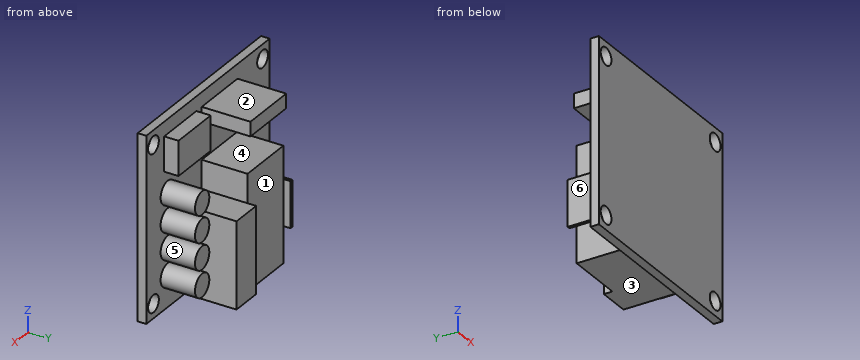
```python
from build123d import *

# Parameters (mm, degrees)
SKETCH_1_W      = 34.5
SKETCH_1_H      = 32
SKETCH_1_R      = 1.5
SKETCH_1_W_2    = 10
SKETCH_1_H_2    = 2.5
SKETCH_1_W_3    = 9
SKETCH_1_H_3    = 6
SKETCH_1_R_2    = 2
SKETCH_1_W_4    = 2.5
SKETCH_1_H_4    = 10
SKETCH_1_W_5    = 0.5
SKETCH_1_H_5    = 8
SKETCH_1_H_6    = 20
SKETCH_1_W_6    = 5.5
SKETCH_1_H_7    = 15
EXTRUDE_1_DEPTH = 1.5
SKETCH_1_3_R    = 2
EXTRUDE_2_DEPTH = 6
SKETCH_1_4_W    = 9
SKETCH_1_4_H    = 6
EXTRUDE_3_DEPTH = 2.5
SKETCH_1_5_W    = 10
SKETCH_1_5_H    = 2.5
EXTRUDE_4_DEPTH = 8.5
SKETCH_1_6_W    = 5.5
SKETCH_1_6_H    = 15
EXTRUDE_5_DEPTH = 9.5
SKETCH_1_7_W    = 10
SKETCH_1_7_H    = 20
EXTRUDE_6_DEPTH = 8
SKETCH_1_9_W    = 0.5
SKETCH_1_9_H    = 8
EXTRUDE_7_DEPTH = 8
SKETCH_1_10_W   = 2.5
SKETCH_1_10_H   = 10
SKETCH_1_10_W_2 = 0.5
SKETCH_1_10_H_2 = 8
EXTRUDE_8_DEPTH = 2.5


with BuildPart() as part:
    # Sketch 1 → Extrude 1 (new body)
    # profile 1 of 11: a face of its own
    with BuildSketch(Plane(origin=(0, 0, 0), x_dir=(1, 0, 0), z_dir=(0, 1, 0))):
        Rectangle(SKETCH_1_W, SKETCH_1_H)
        with Locations(Location((-15.25, -13.5, 0), (0, 0, 270))):
            Circle(SKETCH_1_R, mode=Mode.SUBTRACT)
        with Locations((-3.25, -12.25)):
            Rectangle(SKETCH_1_W_2, SKETCH_1_H_2, mode=Mode.SUBTRACT)
        with Locations((7.75, -10.5)):
            Rectangle(SKETCH_1_W_3, SKETCH_1_H_3, mode=Mode.SUBTRACT)
        with Locations(Location((15.25, -13.5, 0), (0, 0, 270))):
            Circle(SKETCH_1_R, mode=Mode.SUBTRACT)
        with Locations((11.25, -3.5)):
            Circle(SKETCH_1_R_2, mode=Mode.SUBTRACT)
        with Locations((-10.5, 6.5)):
            Rectangle(SKETCH_1_W_4, SKETCH_1_H_4, mode=Mode.SUBTRACT)
        Polygon((-8.25, -4.5), (-8.25, 15.5), (1.75, 15.5), (7.25, 15.5), (7.25, 0.5), (1.75, 0.5), (1.75, -4.5), align=None, mode=Mode.SUBTRACT)
        with Locations(Location((-15.25, 13.5, 0), (0, 0, 270))):
            Circle(SKETCH_1_R, mode=Mode.SUBTRACT)
        with Locations((11.25, 1.166666667)):
            Circle(SKETCH_1_R_2, mode=Mode.SUBTRACT)
        with Locations((11.25, 5.833333333)):
            Circle(SKETCH_1_R_2, mode=Mode.SUBTRACT)
        with Locations((11.25, 10.5)):
            Circle(SKETCH_1_R_2, mode=Mode.SUBTRACT)
        with Locations(Location((15.25, 13.5, 0), (0, 0, 270))):
            Circle(SKETCH_1_R, mode=Mode.SUBTRACT)
    # profile 2 of 11: a face of its own
    with BuildSketch(Plane(origin=(0, 0, 0), x_dir=(1, 0, 0), z_dir=(0, 1, 0))):
        with Locations((-10.5, 6.5)):
            Rectangle(SKETCH_1_W_4, SKETCH_1_H_4)
        with Locations((-10.5, 6.5)):
            Rectangle(SKETCH_1_W_5, SKETCH_1_H_5, mode=Mode.SUBTRACT)
    # profile 3 of 11: a face of its own
    with BuildSketch(Plane(origin=(0, 0, 0), x_dir=(1, 0, 0), z_dir=(0, 1, 0))):
        with Locations((-10.5, 6.5)):
            Rectangle(SKETCH_1_W_5, SKETCH_1_H_5)
    # profile 4 of 11: a face of its own
    with BuildSketch(Plane(origin=(0, 0, 0), x_dir=(1, 0, 0), z_dir=(0, 1, 0))):
        with Locations((-3.25, 5.5)):
            Rectangle(SKETCH_1_W_2, SKETCH_1_H_6)
    # profile 5 of 11: a face of its own
    with BuildSketch(Plane(origin=(0, 0, 0), x_dir=(1, 0, 0), z_dir=(0, 1, 0))):
        with Locations((4.5, 8)):
            Rectangle(SKETCH_1_W_6, SKETCH_1_H_7)
    # profile 6 of 11: a face of its own
    with BuildSketch(Plane(origin=(0, 0, 0), x_dir=(1, 0, 0), z_dir=(0, 1, 0))):
        with Locations((11.25, 10.5)):
            Circle(SKETCH_1_R_2)
    # profile 7 of 11: a face of its own
    with BuildSketch(Plane(origin=(0, 0, 0), x_dir=(1, 0, 0), z_dir=(0, 1, 0))):
        with Locations((11.25, 5.833333333)):
            Circle(SKETCH_1_R_2)
    # profile 8 of 11: a face of its own
    with BuildSketch(Plane(origin=(0, 0, 0), x_dir=(1, 0, 0), z_dir=(0, 1, 0))):
        with Locations((11.25, 1.166666667)):
            Circle(SKETCH_1_R_2)
    # profile 9 of 11: a face of its own
    with BuildSketch(Plane(origin=(0, 0, 0), x_dir=(1, 0, 0), z_dir=(0, 1, 0))):
        with Locations((11.25, -3.5)):
            Circle(SKETCH_1_R_2)
    # profile 10 of 11: a face of its own
    with BuildSketch(Plane(origin=(0, 0, 0), x_dir=(1, 0, 0), z_dir=(0, 1, 0))):
        with Locations((7.75, -10.5)):
            Rectangle(SKETCH_1_W_3, SKETCH_1_H_3)
    # profile 11 of 11: a face of its own
    with BuildSketch(Plane(origin=(0, 0, 0), x_dir=(1, 0, 0), z_dir=(0, 1, 0))):
        with Locations((-3.25, -12.25)):
            Rectangle(SKETCH_1_W_2, SKETCH_1_H_2)
    extrude(amount=-EXTRUDE_1_DEPTH)

    # Sketch 1_3 → Extrude 2 (add)
    with BuildSketch(Plane(origin=(0, 0, 0), x_dir=(1, 0, 0), z_dir=(0, 1, 0))):
        with Locations(Location((11.25, 5.833333333, 0), (0, 0, 270))):
            Circle(SKETCH_1_3_R)
        with Locations(Location((11.25, 10.5, 0), (0, 0, 270))):
            Circle(SKETCH_1_3_R)
        with Locations(Location((11.25, 1.166666667, 0), (0, 0, 270))):
            Circle(SKETCH_1_3_R)
        with Locations(Location((11.25, -3.5, 0), (0, 0, 270))):
            Circle(SKETCH_1_3_R)
    extrude(amount=EXTRUDE_2_DEPTH)

    # Sketch 1_4 → Extrude 3 (add)
    with BuildSketch(Plane(origin=(0, 0, 0), x_dir=(1, 0, 0), z_dir=(0, 1, 0))):
        with Locations((7.75, -10.5)):
            Rectangle(SKETCH_1_4_W, SKETCH_1_4_H)
    extrude(amount=EXTRUDE_3_DEPTH)

    # Sketch 1_5 → Extrude 4 (add)
    with BuildSketch(Plane(origin=(0, 0, 0), x_dir=(1, 0, 0), z_dir=(0, 1, 0))):
        with Locations((-3.25, -12.25)):
            Rectangle(SKETCH_1_5_W, SKETCH_1_5_H)
    extrude(amount=EXTRUDE_4_DEPTH)

    # Sketch 1_6 → Extrude 5 (add)
    with BuildSketch(Plane(origin=(0, 0, 0), x_dir=(1, 0, 0), z_dir=(0, 1, 0))):
        with Locations((4.5, 8)):
            Rectangle(SKETCH_1_6_W, SKETCH_1_6_H)
    extrude(amount=EXTRUDE_5_DEPTH)

    # Sketch 1_7 → Extrude 6 (add)
    with BuildSketch(Plane(origin=(0, 0, 0), x_dir=(1, 0, 0), z_dir=(0, 1, 0))):
        with Locations((-3.25, 5.5)):
            Rectangle(SKETCH_1_7_W, SKETCH_1_7_H)
    extrude(amount=EXTRUDE_6_DEPTH)

    # Sketch 1_9 → Extrude 7 (add)
    with BuildSketch(Plane(origin=(0, 0, 0), x_dir=(1, 0, 0), z_dir=(0, 1, 0))):
        with Locations((-10.5, 6.5)):
            Rectangle(SKETCH_1_9_W, SKETCH_1_9_H)
    extrude(amount=EXTRUDE_7_DEPTH)

    # Sketch 1_10 → Extrude 8 (add)
    with BuildSketch(Plane(origin=(0, 0, 0), x_dir=(1, 0, 0), z_dir=(0, 1, 0))):
        with Locations((-10.5, 6.5)):
            Rectangle(SKETCH_1_10_W, SKETCH_1_10_H)
        with Locations((-10.5, 6.5)):
            Rectangle(SKETCH_1_10_W_2, SKETCH_1_10_H_2, mode=Mode.SUBTRACT)
    extrude(amount=EXTRUDE_8_DEPTH)


solid = part.part
```
Source: CAD feature listing. Evaluate the final solid. Frame: model axes, mm. Face numbers are marked on the shaded views. A direction names the side the tool comes from. Round coordinates to 2 decimals unless told otherwise and drop trailing zeros. Write each loop counter-clockwise with the first axis right and the second up, starting at its lowest first coordinate (ties: lowest second). Pieces come first, ordered by that corner, then holes. Notation, with made-up numbers: M 22,1.5 L 72,1.5 A12 cw 72,24.5 Z; hole C -23.75,-20 d9. An arc over 180 degrees is marked long. Use CSV: the item, a comma, the result in double quotes. Start each with the question number.
Q1. Cut plane C-C on z = -13.5. Output: boundary loops of the cut face in (x, y).
Q2. Line query: line 1 (X direction, y = -0.35, z = -13.5); line 2 (Z direction, x = -6.5, y = 4); line 3 (X direction, y = -0.25, z = -12.5). Output: solid intervals per line, ascending. Write a range as from..to.
Q3. Cut plane D-D on x = -7.5. Output: boundary loops of the cut face in (y, z), plus the area to 3 significant figures.
Q4. First-contact query: P1, Ø3, axis at x = 13.5, y = 3, coming from the +Z side; P2, Ø4, axis at y = 5.5, z = 1.5, coming from the +X side; P3, Ø4, axis at x = -3.5, y = 5.5, coming from the -Z side. Flat tips, straight axial feed; report the tip coordinate or a pass-through.
Q5. Pull-direction query (X, two-part tool) for the marked faces 4, 5 and 6; classes: +X half, -X half, draft (parallel to the pull), parting line (faces both ways), or undercut.
Q6. Cut plane A-A on y = 1.5. Output: boundary loops of the cut face in (x, z).
Q7. Cut plane B-B on x = 15.25. Output: boundary loops of the cut face in (y, z).
Q8. Access query for the marked faces 1, 2 and 3. Directions: +Z, -Z, +X, -X, +Y, -Y. A direction counts if a zero-diameter tool reaches every point of the face in a straight line with its end or side. Return the directions, or none.
Results found:
1,outline,"M -17.25,-1.5 L -16.75,-1.5 L -16.75,0 L -17.25,0 Z; M -13.75,-1.5 L 13.75,-1.5 L 13.75,0 L 7.25,0 L 7.25,9.5 L 1.75,9.5 L 1.75,8 L -8.25,8 L -8.25,0 L -13.75,0 Z; M 16.75,-1.5 L 17.25,-1.5 L 17.25,0 L 16.75,0 Z"
2,line 1,"-17.25..-16.75, -13.75..13.75, 16.75..17.25"
2,line 2,"-15.5..4.5, 11..13.5"
2,line 3,"-17.25..-16.37, -14.13..14.13, 16.37..17.25"
3,outline,"M -1.5,-16 L 0,-16 L 0,-15.5 L 8,-15.5 L 8,4.5 L 0,4.5 L 0,11 L 8.5,11 L 8.5,13.5 L 0,13.5 L 0,16 L -1.5,16 Z"
3,area,"229 mm^2"
4,P1,"z = 13.5"
4,P2,"x = 13.25"
4,P3,"z = -15.5"
5,face 4,"draft"
5,face 5,"undercut"
5,face 6,"-X half"
6,outline,"M -11.75,-11.5 L -9.25,-11.5 L -9.25,-1.5 L -11.75,-1.5 Z; M -8.25,-15.5 L 7.25,-15.5 L 7.25,-0.5 L 1.75,-0.5 L 1.75,4.5 L -8.25,4.5 Z; M -8.25,11 L 1.75,11 L 1.75,13.5 L -8.25,13.5 Z; M 3.25,7.5 L 12.25,7.5 L 12.25,13.5 L 3.25,13.5 Z; C 11.25,-10.5 d4; C 11.25,-5.83 d4; C 11.25,-1.17 d4; C 11.25,3.5 d4"
7,outline,"M -1.5,-16 L 0,-16 L 0,-15 L -1.5,-15 Z; M -1.5,-12 L 0,-12 L 0,12 L -1.5,12 Z; M -1.5,15 L 0,15 L 0,16 L -1.5,16 Z"
8,face 1,"-Z, -X, +Y"
8,face 2,"+Z, +X, -X, +Y"
8,face 3,"-Z, +X, -X, +Y"
